The listing builds one solid part. Answer for the finished solid, in the listing's coordinates (mm). Face numbers are marked on the shaded views. A direction names the side the tool comes from. Give positions to 0.01 mm unless a question says otherwise; leave off trailing zeros. Order: outer loops, then holes, each group sorted by start corner. A loop starts at its lowest first (then second) coordinate and runs counter-clockwise, first axis right, second up. Notation, with made-up numbers: (82.25, -20) - (97.25, -20) arc R15 ccw to (97.25, -1) - close; hole circle Ø2 at (63, 32). An arc over 180 degrees is marked (long way). Answer as CSV lines item,"result". Start each with the question number.
1. Consider line 1 along Z through (x, y) = (0.5, 0); line 2 along X through (y, z) = (-1.55, 1.3); line 3 along Y through (x, z) = (4.75, 0.7). Determine where each line is inside the solid, lowest interval first. Write a range as [from, to].
2. Which of the six approach directions +Z, -Z, +X, -X, +Y, -Y give full straight-line access (tool end or side, diameter ignored) to the marked faces 1 and 2?
3. A flat-ended cylindrical pin translates along its axis: pin 1 (1 mm diameter, centred on x = -1, y = 2, fed in from +Z). Find the tip coordinate at first contact, or state that the pin passes through.
4. Determine the mould class of the marked faces 3, 4 and 5 for opening direction Z: +Z half, -Z half, draft (parallel to the pull), parting line (faces both ways), or undercut.
5. Section A-A on x = 6.5 is taken. Give the vertices of the cut face in (y, z), and give its area (3 significant figures).
Autodesk Inventor part; units mm, degrees
ref_plane "Work Plane1" through (29, 0, 0) normal (0, -1, 0) x (1, 0, 0)
ref_plane "YZ Plane" through (0, 0, 0) normal (1, 0, 0) x (0, 1, 0)
ref_plane "XZ Plane" through (0, 0, 0) normal (0, 1, 0) x (-1, 0, 0)
sketch "Sketch1" plane through (0, 0, 0) normal (0, 0, 1) x (1, 0, 0)
  line L0 (-0.7535, 0) -> (7.9375, 0)
  line L1 (7.9375, 0) -> (7.9375, 1.4224)
  line L2 (7.9375, 1.4224) -> (2.4448, 1.4224)
  line L3 (2.4448, 1.4224) -> (0.8572, 1.4224)
  line L4 (0.8572, 1.4224) -> (0, 1.4224)
  line L5 (0, 1.4224) -> (0, 2.3241)
  line L6 (0, 2.3241) -> (-2.8448, 2.3241)
  line L7 (-2.8448, 2.3241) -> (-2.8448, 1.3785)
  line L8 (-2.8448, 1.3785) -> (-1.5494, 1.3785)
  line L9 (-1.5494, 1.3785) -> (-0.7535, 0)
  line L10 (-5.0013, 0) -> (10.094, 0)
  line L11 (0, -0.4648) -> (0, 2.7889)
  line L12 (2.4448, 1.4224) -> (0, 1.4224) construction
  dimension "d1" = 5.4928
  dimension "d2" = 1.5876
  dimension "d3" = 2.8448
  dimension "d4" = 1.2954
  dimension "d5" = 60
  dimension "d6" = 2.8448
  dimension "d7" = 2.8448
  dimension "d8" = 2.757
  dimension "d9" = 4.6482
  dimension "d26" = 7.9375
revolve "Body" add sketch "Sketch1" angle 360 about axis through (-0.7535, 0, 0) along (1, 0, 0)
sketch "Sketch2" plane through (-2.8448, 0, 0) normal (-1, 0, 0) x (0, 0, 1)
  circle A0 centre (0, 0) radius 1.3785
  line L0 (0, -3.2537) -> (0, 3.2537)
  line L1 (-3.2537, 0) -> (3.2537, 0)
  line L2 (1.3785, 0) -> (0.6892, -1.1938)
  line L3 (0.6892, -1.1938) -> (-0.6892, -1.1938)
  line L4 (-0.6892, -1.1938) -> (-1.3785, 0)
  line L5 (-1.3785, 0) -> (-0.6892, 1.1938)
  line L6 (-0.6892, 1.1938) -> (0.6892, 1.1938)
  line L7 (0.6892, 1.1938) -> (1.3785, 0)
  point P0 (0, 0)
extrude "Slot" add sketch "Sketch2" against normal up to next contours L7 A0 | A0 L2 | L6 L0 A0 | A0 L0 L3 | L0 L6 A0 | A0 L3 L0 | L4 A0 | A0 L5
fillet "Fillet1" radius 0.2286 1 edges at (-2.8448, -2.3241, 0)
thread "Thread"
chamfer "Chamfer1" distance 0.3785 distance2 0.3785 1 edges at (7.9375, -1.4224, 0) measured on face at (7.9375, -0.3549, 0.3144)
ref_plane "Work Plane1" through (29, 0, 0) normal (0, -1, 0) x (1, 0, 0)
fillet "Fillet2" radius 0.1016 1 edges at (0, -1.4224, 0)
equation "\"d1\" = GEL"
equation "\"d3\" = KOH"
equation "\"d4\" = INTI"
equation "\"d6\" = GD"
equation "\"d7\" = BDM"
equation "\"d8\" = 1.1547 * SW"
equation "\"d9\" = KOD"
equation "\"d26\" = NLG"
equation "\"d30\" = R"
equation "\"d17\" = RR"
equation "\"d13\" = GEL"
equation "\"d15\" = -0.5 * SPD + 0.5 * GD"
equation "\"d16\" = GUL"
equation "\"GD\" = 2.8448"
equation "\"NLG\" = 7.9375"
equation "\"GEL\" = 5.49275"
equation "\"KOD\" = 4.6482"
equation "\"KOH\" = 2.8448"
equation "\"INTI\" = 1.2954"
equation "\"GAL\" = 1.5875"
equation "\"GUL\" = 0.37846"
equation "\"BDM\" = 2.8448"
equation "\"SW\" = 2.3876"
equation "\"RR\" = 0.2286"
equation "\"SPD\" = 2.08788"
equation "\"R\" = 0.1016"
equation "\"PHH\" = 0.127"
equation "\"GD1\" = SPD"
equation "\"THREADDIA\" = 2.8448"
equation "\"FAWI\" = 45deg"
equation "\"KOH1\" = 2.5654"
equation "\"NND\" = 2.8448"
equation "\"TOA\" = 30deg"
equation "\"E0\" = 1.155 * SW"
properties part number "ANSI B18.3 - No. 4 - 40 UNC - 5/16 HS HCS" material "Steel, Alloy"
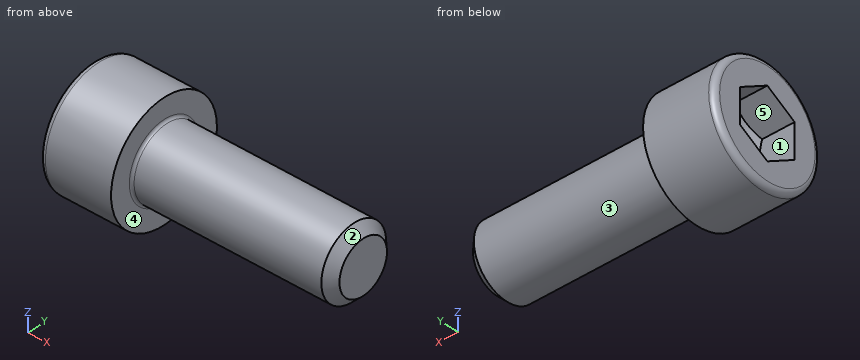
Checks:
1,line 1,"z = [-1.42, 1.42]"
1,line 2,"x = [-2.84, 0]"
1,line 3,"y = [-1.24, 1.24]"
2,face 1,"-X"
2,face 2,"+X"
3,pin 1,"stops at z = 1.78"
4,face 3,"parting line"
4,face 4,"draft"
4,face 5,"undercut"
5,outline,"circle Ø2.84 at (0, 0)"
5,area,"6.36 mm²"
